from build123d import *

# Parameters (mm, degrees)
SCHIZZO1_R                   = 4
ESTRUSIONE_ESTRUSIONE1_DEPTH = 8
SMUSSO1_SIZE                 = 1
SCHIZZO6_R                   = 5
ESTRUSIONE_ESTRUSIONE3_DEPTH = 6
TAGLIO_ESTRUSIONE3_DEPTH     = 3
SCHIZZO8_R                   = 2.886751346
TAGLIO_ESTRUSIONE4_DEPTH     = 1
TAGLIO_ESTRUSIONE4_TAPER     = 45
RACCORDO1_R                  = 0.23
RACCORDO2_R                  = 0.2


with BuildPart() as part:
    # Schizzo1 → Estrusione-Estrusione1 (new body)
    with BuildSketch(Plane.XY):
        Circle(SCHIZZO1_R)
    extrude(amount=ESTRUSIONE_ESTRUSIONE1_DEPTH)

    # Smusso1
    smusso1_edges = [part.edges().sort_by_distance(p)[0] for p in [
        (-4, 0, 0),
    ]]
    chamfer(smusso1_edges, length=SMUSSO1_SIZE)

    # Schizzo6 → Estrusione-Estrusione3 (add)
    with BuildSketch(Plane.XY.offset(8)):
        Circle(SCHIZZO6_R)
    extrude(amount=ESTRUSIONE_ESTRUSIONE3_DEPTH)

    # Schizzo7 → Taglio-Estrusione3 (cut)
    with BuildSketch(Plane.XY.offset(14)):
        Polygon((1.443375673, 2.5), (-1.443375673, 2.5), (-2.886751346, 0), (-1.443375673, -2.5), (1.443375673, -2.5), (2.886751346, 0), align=None)
    extrude(amount=-TAGLIO_ESTRUSIONE3_DEPTH, mode=Mode.SUBTRACT)

    # Schizzo8 → Taglio-Estrusione4 (cut)
    with BuildSketch(Plane.XY.offset(14)):
        Circle(SCHIZZO8_R)
    extrude(amount=-TAGLIO_ESTRUSIONE4_DEPTH, taper=TAGLIO_ESTRUSIONE4_TAPER, mode=Mode.SUBTRACT)

    # Raccordo1
    raccordo1_edges = [part.edges().sort_by_distance(p)[0] for p in [
        (-5, 0, 14),
    ]]
    fillet(raccordo1_edges, radius=RACCORDO1_R)

    # Raccordo2
    raccordo2_edges = [part.edges().sort_by_distance(p)[0] for p in [
        (-5, 0, 8),
    ]]
    fillet(raccordo2_edges, radius=RACCORDO2_R)


solid = part.part
The model under review builds one solid part; all positions refer to its coordinate system, in mm. A direction names the side the tool comes from. Give positions to 0.01 mm unless a question says otherwise; leave off trailing zeros. Loops run counter-clockwise (first coordinate to the right, second up) from the corner with the lowest first, then second, coordinate; pieces in that order, holes last. Notation, with made-up numbers: (-1, -32.5) -> (46, -32.5) arc R12 ccw to (46, -21.5) -> close; hole circle Ø9 at (89.5, 77.25). An arc over 180 degrees is marked (long way). Answer as a JSON object with one key per item and string values. Group by question number.
Q1. Take a section at C-C (z = 3). Write out the cut boundary in (x, y).
Q2. Wall thickness on line 1 along Z through (x, y) = (2.5, -3.25); line 2 along Z through (x, y) = (-1, 0.75); line 3 along Y through (x, z) = (-4, 11.25): over which ranges is each line inside the solid? List them lowest first.
Q3. Insertion check: pin 1 (1.5 mm diameter, centred on x = -2.5, y = 4, fed in from -Z); pin 2 (1.5 mm diameter, centred on x = 1, y = 0.5, fed in from +Z); pin 3 (1 mm diameter, centred on y = 3, z = 6.5, fed in from -X). Each pin has a flat end and moves straight along its axis. Give the tip position at first contact, or say it passes through.
Q4. Tool access review of faces 1 (the flat face through (-0.1, -3.1, 14)), 2 (the conical face through (-2.34, -1.328, 13.804)): name each direction out of +Z, -Z, +X, -X, +Y, -Y from which nothing blocks a thin tool from reaching the whole face with its end or side.
Q5. Take a section at A-A (x = 0). Write out the cut boundary in (y, z).
Q6. Take a section at B-B (z = 12). Write out the cut boundary in (x, y), plus the area to 3 significant figures.
Q7. Draft analysis for pull direction Y (two halves, no side actions). For faces 3 (the flat face through (-2, 4, 8)), 4 (the cylindrical face through (-0.867, -3.905, 4.451)), 5 (the flat face through (0, -2.5, 13)), state which applies: pulls with the +Y half, pulls with the -Y half, needs draft (parallel to the pull), parting line crosses it, or undercut.
Answer below:
{
 "1": {"outline": "circle Ø8 at (0, 0)"},
 "2": {"line 1": "z = 8 to 14", "line 2": "z = 0 to 11", "line 3": "y = -3 to 3"},
 "3": {"pin 1": "stops at z = 0.97", "pin 2": "stops at z = 11", "pin 3": "stops at x = -3.12"},
 "4": {"face 1": "+Z, +X, -X, +Y, -Y", "face 2": "+Z"},
 "5": {"outline": "(-5, 8.2) arc R0.2 ccw to (-4.8, 8) -> (-4, 8) -> (-4, 1) -> (-3, 0) -> (3, 0) -> (4, 1) -> (4, 8) -> (4.8, 8) arc R0.2 ccw to (5, 8.2) -> (5, 13.77) arc R0.23 ccw to (4.77, 14) -> (2.89, 14) -> (2.5, 13.61) -> (2.5, 11) -> (-2.5, 11) -> (-2.5, 13.61) -> (-2.89, 14) -> (-4.77, 14) arc R0.23 ccw to (-5, 13.77) -> close"},
 "6": {"outline": "circle Ø10 at (0, 0); hole (-2.89, 0) -> (-1.44, -2.5) -> (1.44, -2.5) -> (2.89, 0) -> (1.44, 2.5) -> (-1.44, 2.5) -> close", "area": "56.9 mm2"},
 "7": {"face 3": "needs draft", "face 4": "parting line crosses it", "face 5": "undercut"}
}
